Work out the finished part from the listing and answer in its coordinate system (mm). Face numbers are marked on the shaded views. A direction names the side the tool comes from. Round coordinates to 2 decimals unless told otherwise and drop trailing zeros. Write each loop counter-clockwise with the first axis right and the second up, starting at its lowest first coordinate (ties: lowest second). Pieces come first, ordered by that corner, then holes. Notation, with made-up numbers: (81.5, 74.25) -> (113.5, 74.25) arc R25 cw to (113.5, 109.25) -> close; hole circle Ø4 at (-18.5, 89). An arc over 180 degrees is marked (long way). One line per item, written item: value.
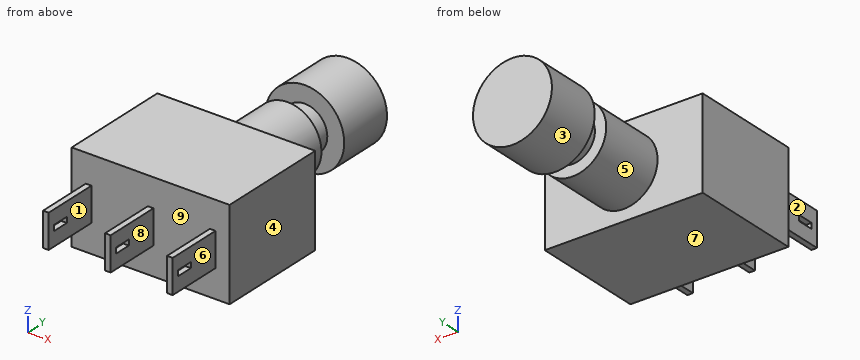
```python
from build123d import *

# Parameters (mm, degrees)
SKETCH2_W          = 14
SKETCH2_H          = 8
EXTRUDE1_DEPTH     = 10
SKETCH3_R          = 3
EXTRUDE2_DEPTH     = 6
SKETCH4_R          = 2
EXTRUDE3_DEPTH     = 2
SKETCH5_R          = 3.5
EXTRUDE4_DEPTH     = 5
SKETCH6_W          = 0.5
SKETCH6_H          = 3
EXTRUDE5_DEPTH     = 5
SKETCH7_W          = 0.5
SKETCH7_H          = 3
EXTRUDE6_DEPTH     = 5
SKETCH8_W          = 0.5
SKETCH8_H          = 3
EXTRUDE7_DEPTH     = 5
SKETCH9_W          = 0.5
SKETCH9_H          = 1.5
CUT_EXTRUDE1_DEPTH = 27.600046992


with BuildPart() as part:
    # Sketch2 → Extrude1 (new body)
    with BuildSketch(Plane(origin=(0, 0, 0), x_dir=(1, 0, 0), z_dir=(0, 1, 0))):
        Rectangle(SKETCH2_W, SKETCH2_H)
    extrude(amount=EXTRUDE1_DEPTH)

    # Sketch3 → Extrude2 (add)
    with BuildSketch(Plane(origin=(0, 10, 0), x_dir=(-1, 0, 0), z_dir=(0, 1, 0))):
        with Locations(Location((0, 0, 0), (0, 0, 90))):
            Circle(SKETCH3_R)
    extrude(amount=EXTRUDE2_DEPTH)

    # Sketch4 → Extrude3 (add)
    with BuildSketch(Plane(origin=(0, 16, 0), x_dir=(-1, 0, 0), z_dir=(0, 1, 0))):
        with Locations(Location((0, 0, 0), (0, 0, 90))):
            Circle(SKETCH4_R)
    extrude(amount=EXTRUDE3_DEPTH)

    # Sketch5 → Extrude4 (add)
    with BuildSketch(Plane(origin=(0, 18, 0), x_dir=(-1, 0, 0), z_dir=(0, 1, 0))):
        with Locations(Location((0, 0, 0), (0, 0, 90))):
            Circle(SKETCH5_R)
    extrude(amount=EXTRUDE4_DEPTH)

    # Sketch6 → Extrude5 (add)
    with BuildSketch(Plane.XZ):
        Rectangle(SKETCH6_W, SKETCH6_H)
    extrude(amount=EXTRUDE5_DEPTH)

    # Sketch7 → Extrude6 (add)
    with BuildSketch(Plane.XZ):
        with Locations((5.5, 0)):
            Rectangle(SKETCH7_W, SKETCH7_H)
    extrude(amount=EXTRUDE6_DEPTH)

    # Sketch8 → Extrude7 (add)
    with BuildSketch(Plane.XZ):
        with Locations((-5.5, 0)):
            Rectangle(SKETCH8_W, SKETCH8_H)
    extrude(amount=EXTRUDE7_DEPTH)

    # Sketch9 → Cut-Extrude1 (cut, through all)
    with BuildSketch(Plane.ZY.offset(5.75)):
        with Locations((0, -3.626725107)):
            Rectangle(SKETCH9_W, SKETCH9_H)
    extrude(amount=-CUT_EXTRUDE1_DEPTH, mode=Mode.SUBTRACT)


solid = part.part
```
(1) Find section B-B on z = 2.5. Give the vertices of the cut face in (x, y), plus the area to 3 significant figures.
Reported:
outline: (-7, 0) -> (7, 0) -> (7, 10) -> (1.66, 10) -> (1.66, 16) -> (-1.66, 16) -> (-1.66, 10) -> (-7, 10) -> close; (-2.45, 18) -> (2.45, 18) -> (2.45, 23) -> (-2.45, 23) -> close
area: 184 mm2
(2) Find section C-C on x = -2.5. Give the vertices of the cut face in (y, z), plus the area to 3 significant figures.
Reported:
outline: (0, -4) -> (10, -4) -> (10, -1.66) -> (16, -1.66) -> (16, 1.66) -> (10, 1.66) -> (10, 4) -> (0, 4) -> close; (18, -2.45) -> (23, -2.45) -> (23, 2.45) -> (18, 2.45) -> close
area: 124 mm2
(3) Find section D-D on y = 20. Give the vertices of the cut face in (x, z), plus the area to 3 significant figures.
Reported:
outline: circle Ø7 at (0, 0)
area: 38.5 mm2
(4) Find section A-A on y = -1. Give the vertices of the cut face in (x, z), plus the area to 3 significant figures.
Reported:
outline: (-5.75, -1.5) -> (-5.25, -1.5) -> (-5.25, 1.5) -> (-5.75, 1.5) -> close; (-0.25, -1.5) -> (0.25, -1.5) -> (0.25, 1.5) -> (-0.25, 1.5) -> close; (5.25, -1.5) -> (5.75, -1.5) -> (5.75, 1.5) -> (5.25, 1.5) -> close
area: 4.50 mm2
(5) For a pull along X with two mould halves and no side action, classify the marked faces 6, 7, 8 and 9 as pulls with the +X half, pulls with the -X half, needs draft (parallel to the pull), parting line crosses it, or undercut.
Reported:
face 6: pulls with the +X half
face 7: needs draft
face 8: undercut
face 9: undercut
(6) Consider probe 1 along X at (y, z) = (-0.5, 0); probe 2 along Y at (x, z) = (-1, 3.5); probe 3 along Y at (x, z) = (-1, 2). Determine where each line is inside the solid, lowest interval first.
Reported:
probe 1: x = -5.75 to -5.25, -0.25 to 0.25, 5.25 to 5.75
probe 2: y = 0 to 10
probe 3: y = 0 to 16, 18 to 23
(7) A tool of negligible diameter and unlimited length cuts with its end or side. For the marked faces 1, 2, 3, 4 and 5, from which of +Z, -Z, +X, -X, +Y, -Y can it reach the whole face along a straight path? Write none if from no direction.
Reported:
face 1: +Z, -Z, -Y
face 2: +Z, -Z, -X, -Y
face 3: +Y
face 4: +Z, -Z, +X, +Y, -Y
face 5: none
(8) Flat-ended cylindrical pins translate along their axes: pin 1 Ø0.6 at (x, y) = (-5.5, -3.5) entering from +Z; pin 2 Ø1.5 at (y, z) = (15, 3) entering from +X; pin 3 Ø1.5 at (y, z) = (-2, 0.5) entering from +X. Find the tip coordinate at first contact, or state that the pin passes through.
Reported:
pin 1: stops at z = 1.5
pin 2: stops at x = 1.98
pin 3: stops at x = 5.75
